The model under review builds one solid part; all positions refer to its coordinate system, in mm. A direction names the side the tool comes from. Coordinates: 2 decimals unless noted, no trailing zeros. Write each loop counter-clockwise with the first axis right and the second up, starting at its lowest first coordinate (ties: lowest second). Pieces come first, ordered by that corner, then holes.
```python
from build123d import *

# Parameters (mm, degrees)
F0_W         = 111.8826307356
F0_H         = 33.61280635
F1_DEPTH     = 48
F3_DEPTH     = 92
F5_DEPTH     = 9
F6_T1_DEPTH  = 94.5960432291
F7_R         = 5
F8_R         = 5
F9_R         = 5
F10_T1_DEPTH = 136.8826307356
F10_T3_DEPTH = 127.4671918099


# Not quite as in the source:
# - a fillet or chamfer that OpenCascade refuses, or shapes differently, is made with other operations: its cross-section is extruded or revolved along the edge and cut away or added


with BuildPart() as f1:
    # F0 (on Top) → F1 (new body)
    with BuildSketch(Plane.XY):
        with Locations((-7.0826988667, -28.0907023698)):
            Rectangle(F0_W, F0_H)
    extrude(amount=F1_DEPTH)

    # F2 (on Right) → F3 (cut, symmetric)
    with BuildSketch(Plane.YZ):
        Polygon((-2.2725867394, 56.280748791), (-39.9752296507, 54.2606711388), (-27.7305655181, 29.2911604047), (-4.6817823313, 27.3704268038), align=None)
    extrude(amount=F3_DEPTH, both=True, mode=Mode.SUBTRACT)

    # F4 (on face) → F5 (cut)
    with BuildSketch(Plane(origin=(0, 2.2328525009, 26.7942067339), x_dir=(1, 0, 0), z_dir=(0, 0.0830455515, 0.9965457523))):
        Polygon((40.2153246105, -5.8544473723), (-54.3807186186, -8.7455315515), (-54.3807186186, -30.0672778452), (40.2153246105, -30.0672778452), align=None)
    extrude(amount=-F5_DEPTH, mode=Mode.SUBTRACT)

    # F6: fillet of radius 53.3943165321 on 1 edges, made by hand

    # F6_s2 → F6_t1 (cut)
    with BuildSketch(Plane.YZ.offset(-54.3807186186)):
        with BuildLine():
            ThreePointArc((-33.8957137688, 41.863227205), (-30.0543394398, 31.3775725516), (-28.4779754817, 20.3222486342))
            Line((-28.4779754817, 20.3222486342), (-27.7305655181, 29.2911604047))
            Line((-27.7305655181, 29.2911604047), (-33.8957137688, 41.863227205))
        make_face()
    extrude(amount=F6_T1_DEPTH, mode=Mode.SUBTRACT)

    # F7
    f7_edges = [f1.edges().sort_by_distance(p)[0] for p in [
        (-54.380719, -19.507432, 28.605899),
        (40.215325, -19.507432, 28.605899),
    ]]
    fillet(f7_edges, radius=F7_R)

    # F8
    f8_edges = [f1.edges().sort_by_distance(p)[0] for p in [
        (-7.082697, -11.284299, 18.889441),
    ]]
    fillet(f8_edges, radius=F8_R)

    # F9
    f9_edges = [f1.edges().sort_by_distance(p)[0] for p in [
        (-63.024014, -28.090702, 0),
        (48.858617, -28.090702, 0),
    ]]
    fillet(f9_edges, radius=F9_R)

    # F10: fillet of radius 5 on 2 edges, made by hand

    # F10_s2 → F10_t1 (cut)
    with BuildSketch(Plane.YZ.offset(-75.5240142345)):
        with BuildLine():
            ThreePointArc((-44.8971055448, 43), (-43.4326394507, 46.5355339059), (-39.8971055448, 48))
            Line((-39.8971055448, 48), (-44.8971055448, 48))
            Line((-44.8971055448, 48), (-44.8971055448, 43))
        make_face()
    extrude(amount=F10_T1_DEPTH, mode=Mode.SUBTRACT)

    # F10_s4 → F10_t3 (cut)
    with BuildSketch(Plane.YZ.offset(-70.8162947717)):
        with BuildLine():
            ThreePointArc((-35.5327359736, 45.2014685051), (-37.3769475866, 47.2430733275), (-40.0220050033, 48))
            Line((-40.0220050033, 48), (-36.9050927884, 48))
            Line((-36.9050927884, 48), (-35.5327359736, 45.2014685051))
        make_face()
    extrude(amount=F10_T3_DEPTH, mode=Mode.SUBTRACT)


solid = f1.part
```
Item 1: Take a section at C-C, the plane y = -31. Write out the cut boundary in (x, z).
Solved:
outline: (-63.02, 5) arc R5 ccw to (-58.02, 0) - (43.86, 0) arc R5 ccw to (48.86, 5) - (48.86, 35.96) - (40.22, 35.96) - (40.22, 34.68) - (-54.38, 34.68) - (-54.38, 35.96) - (-63.02, 35.96) - close
Item 2: Take a section at B-B, the plane z = 31. Write out the cut boundary in (x, y).
Solved:
outline: (-63.02, -44.9) - (48.86, -44.9) - (48.86, -28.57) - (40.22, -28.57) - (40.22, -29.96) - (-54.38, -29.96) - (-54.38, -28.57) - (-63.02, -28.57) - close
Item 3: For pin 1 (1 mm diameter, centred on x = 37, z = 31.5, fed in from +Y), flat-tipped, find the tip position at first contact; note if it passes through.
Solved:
pin 1: stops at y = -29.96
Item 4: Machinability: for faces 5 (the face through (-7.74, -22.09, 19.79)), 6 (the face through (-8, -11.284, 11)), which of the approach directions +Z, -Z, +X, -X, +Y, -Y give a long, thin tool a straight path to every point of the face, cutting with its end or side? Answer none if there is none.
Solved:
face 5: +Z, +Y
face 6: +Z, -Z, +X, -X, +Y
Item 5: To check wall thickness, follow line 1 along Y through (x, z) = (-49.5, 35); line 2 along Z through (x, y) = (40, -25); line 3 along Z through (x, y) = (29, -34). State the ranges of each line that lie inside material, in increasing order.
Solved:
line 1: y = -44.9 to -31.1
line 2: z = 0 to 20.03
line 3: z = 0 to 42.08
Item 6: Mouldability with a two-part tool opening along X and no side actions: class faces 1 (the face through (-6.421, -12.57, 17.636)), 2 (the face through (47.36, -27.86, 1.43)), 3 (the face through (-54.381, -21, 23)), 4 (the face through (-61.598, -27.855, 1.504)) as pulls with the +X half, pulls with the -X half, needs draft (parallel to the pull), parting line crosses it, or undercut.
Solved:
face 1: undercut
face 2: pulls with the +X half
face 3: undercut
face 4: pulls with the -X half
Item 7: Take a section at D-D, the plane z = 37.5. Write out the cut boundary in (x, y).
Solved:
outline: (-63.02, -44.9) - (48.86, -44.9) - (48.86, -31.76) - (40.22, -31.76) - (40.22, -31.99) - (-54.38, -31.99) - (-54.38, -31.76) - (-63.02, -31.76) - close
Item 8: Take a section at A-A, the plane x = -11.5. Write out the cut boundary in (y, z).
Solved:
outline: (-44.9, 0) - (-11.28, 0) - (-11.28, 14.29) arc R5 ccw to (-15.87, 19.27) - (-28.48, 20.32) arc R53.39 ccw to (-33.9, 41.86) - (-35.53, 45.2) arc R5 ccw to (-39.96, 48) arc R5 ccw to (-44.9, 43) - close
